Verification items for the finished model (mm, model axes). A direction names the side the tool comes from. Round coordinates to 2 decimals unless told otherwise and drop trailing zeros. Write each loop counter-clockwise with the first axis right and the second up, starting at its lowest first coordinate (ties: lowest second). Pieces come first, ordered by that corner, then holes.
from build123d import *

# Parameters (mm, degrees)
SKETCH1_W           = 75
SKETCH1_H           = 12
SKETCH1_R           = 17.5
SKETCH1_R_2         = 11
BOSS_EXTRUDE1_DEPTH = 10
FILLET1_R           = 4
FILLET2_R           = 12


with BuildPart() as part:
    # Sketch1 → Boss-Extrude1 (new body)
    with BuildSketch(Plane(origin=(0, 0, 0), x_dir=(1, 0, 0), z_dir=(0, 1, 0))):
        with BuildLine():
            Line((197.072466256, 12), (12.737739203, 12))
            ThreePointArc((12.737739203, 12), (16.265921985, 6.45521355), (17.5, 0))
            ThreePointArc((17.5, 0), (16.265921985, -6.45521355), (12.737739203, -12))
            Line((12.737739203, -12), (207.262260797, -12))
            ThreePointArc((207.262260797, -12), (202.5, 0), (207.262260797, 12))
            Line((207.262260797, 12), (197.072466256, 12))
        make_face()
        with Locations((65, 0)):
            Rectangle(SKETCH1_W, SKETCH1_H, mode=Mode.SUBTRACT)
        with Locations((155, 0)):
            Rectangle(SKETCH1_W, SKETCH1_H, mode=Mode.SUBTRACT)
        Circle(SKETCH1_R)
        Circle(SKETCH1_R_2, mode=Mode.SUBTRACT)
        with Locations((220, 0)):
            Circle(SKETCH1_R)
        with Locations((220, 0)):
            Circle(SKETCH1_R_2, mode=Mode.SUBTRACT)
    extrude(amount=BOSS_EXTRUDE1_DEPTH)

    # Fillet1
    fillet1_edges = [part.edges().sort_by_distance(p)[0] for p in [
        (27.5, 5, -6),
        (27.5, 5, 6),
        (102.5, 5, 6),
        (102.5, 5, -6),
        (117.5, 5, -6),
        (117.5, 5, 6),
        (192.5, 5, 6),
        (192.5, 5, -6),
    ]]
    fillet(fillet1_edges, radius=FILLET1_R)

    # Fillet2
    fillet2_edges = [part.edges().sort_by_distance(p)[0] for p in [
        (12.737739203, 5, 12),
        (12.737739203, 5, -12),
        (207.262260797, 5, -12),
        (207.262260797, 5, 12),
    ]]
    fillet(fillet2_edges, radius=FILLET2_R)


solid = part.part
Q1. Sectioned sample at C-C (x = 220). Enter the section's corners in (y, z).
Recorded:
outline: (0, -17.5) - (10, -17.5) - (10, -11) - (0, -11) - close; (0, 11) - (10, 11) - (10, 17.5) - (0, 17.5) - close
Q2. Depth check by flat-ended pin: P1, Ø5, axis at x = 77.5, y = 7, coming from the -Z side; P2, Ø6, axis at x = 91.5, y = 8, coming from the +Z side; P3, Ø1, axis at y = 4, z = 8, coming from the +X side; P4, Ø20, axis at x = 0, z = 0, coming from the -Y side. Enter the tip coordinate at first touch or a pass-through.
Recorded:
P1: stops at z = -12
P2: stops at z = 12
P3: stops at x = 235.81
P4: passes through
Q3. Material ranges on line 1 along X through (y, z) = (4.75, -0.5); line 2 along Z through (x, y) = (173, 3); line 3 along Z through (x, y) = (0, 3), recorded low to high.
Recorded:
line 1: x = -17.49 to -10.99, 10.99 to 27.5, 102.5 to 117.5, 192.5 to 209.01, 230.99 to 237.49
line 2: z = -12 to -6, 6 to 12
line 3: z = -17.5 to -11, 11 to 17.5
Q4. Release check for a two-part mould opening along X. For faces 4 (the flat face through (108, 0, 0)), 5 (the flat face through (117.5, 5, 0)) record: released by +X, released by -X, zero draft, split by the parting line, or undercut.
Recorded:
face 4: zero draft
face 5: undercut
Q5. Tool access check on faces 1 (the cylindrical face through (28.641, 5.07, -4.797)), 2 (the flat face through (109, 5, 12)), 3 (the cylindrical face through (206.46, 5.07, -12.557)). Record the directions out of +Z, -Z, +X, -X, +Y, -Y that give a thin tool (end or side, any length) a straight path to the whole face; none if there is none.
Recorded:
face 1: +Y, -Y
face 2: +Z, +Y, -Y
face 3: -Z, +Y, -Y
Q6. Sectioned sample at B-B (y = 2.5). Enter the section's corners in (x, z), plus the area to 3 significant figures.
Recorded:
outline: (10.18, -14.24) arc R12 cw to (17.15, -12) - (202.85, -12) arc R12 cw to (209.82, -14.24) arc R17.5 ccw (long way) to (209.82, 14.24) arc R12 cw to (202.85, 12) - (17.15, 12) arc R12 cw to (10.18, 14.24) arc R17.5 ccw (long way) to start; hole circle Ø22 at (0, 0); hole (27.5, -2) arc R4 ccw to (31.5, -6) - (98.5, -6) arc R4 ccw to (102.5, -2) - (102.5, 2) arc R4 ccw to (98.5, 6) - (31.5, 6) arc R4 ccw to (27.5, 2) - close; hole (117.5, -2) arc R4 ccw to (121.5, -6) - (188.5, -6) arc R4 ccw to (192.5, -2) - (192.5, 2) arc R4 ccw to (188.5, 6) - (121.5, 6) arc R4 ccw to (117.5, 2) - close; hole circle Ø22 at (220, 0)
area: 3,910 mm2
Q7. Sectioned sample at A-A (x = 161.5). Enter the section's corners in (y, z), plus the area to 3 significant figures.
Recorded:
outline: (0, -12) - (10, -12) - (10, -6) - (0, -6) - close; (0, 6) - (10, 6) - (10, 12) - (0, 12) - close
area: 120 mm2
